Design review of the part built by this model. Coordinates are the model's own, in mm. A direction names the side the tool comes from. Coordinates: 2 decimals unless noted, no trailing zeros. Write each loop counter-clockwise with the first axis right and the second up, starting at its lowest first coordinate (ties: lowest second). Pieces come first, ordered by that corner, then holes.
Q1. Mouldability with a two-part tool opening along Y and no side actions: class faces 1 (the flat face through (-1.6, -9.5, -88.816)), 2 (the flat face through (-1, -15, -104)), 3 (the flat face through (-1, 170, 1)) as pulls with the +Y half, pulls with the -Y half, needs draft (parallel to the pull), parting line crosses it, or undercut.
Q2. For probe 1 along Y at (x, z) = (-41.5, 36); probe 2 along Z at (x, y) = (0, 85.5); probe 3 along Z at (x, y) = (88, -4.5), list the stretches that pass through material, from the lowest coordinate up.
Q3. Take a section at B-B (y = 131). Give the boundary of the cut face in (x, z), and give its area (3 significant figures).
Q4. Take a section at D-D (x = 90.5). Give the boundary of the cut face in (y, z), and give its area (3 significant figures).
Q5. Take a section at C-C (z = 49). Give the boundary of the cut face in (x, y), and give its area (3 significant figures).
Q6. Take a section at A-A (x = 0). Give the boundary of the cut face in (y, z), and give its area (3 significant figures).
Q7. Insertion check: pin 1 (10 mm diameter, centred on x = 46, y = 2.5, fed in from +Z); pin 2 (4 mm diameter, centred on x = -31, y = 138, fed in from -Z); pin 3 (20.5 mm diameter, centred on x = 4.5, z = -101, fed in from -Y). Each pin has a flat end and moves straight along its axis. Give the tip position at first contact, or say it passes through.
Q8. Machinability: for faces 4 (the flat face through (-2, -25, -18)), 5 (the conical face through (40.05, 86.19, 12.61)), 6 (the flat face through (-1, -10, -104)), which of the approach directions +Z, -Z, +X, -X, +Y, -Y give a long, thin tool a straight path to every point of the face, cutting with its end or side? Answer none if there is none.
```python
from build123d import *

# Parameters (mm, degrees)
F0_R     = 45
F1_DEPTH = 170
F1_TAPER = 2
F3_DEPTH = 25
F5_START = -10
F4_R     = 92.5
F5_DEPTH = 5


with BuildPart() as f1:
    # F0 (on Front) → F1 (new body)
    with BuildSketch(Plane.XZ):
        Circle(F0_R)
    extrude(amount=-F1_DEPTH, taper=F1_TAPER)

    # F2 (on face) → F3 (join)
    with BuildSketch(Plane.XZ):
        with BuildLine():
            Line((-114.8654392336, -88.8156135872), (114.8654392336, -88.8156135872))
            ThreePointArc((114.8654392336, -88.8156135872), (0, 89.0399508403), (-114.8654392336, -88.8156135872))
        make_face()
    extrude(amount=F3_DEPTH)

    # F4 (on face) → F5 (join)
    with BuildSketch(Plane.XZ.offset(25).offset(F5_START)):
        with Locations((0, -36.9799211621)):
            Circle(F4_R)
    extrude(amount=-F5_DEPTH)


solid = f1.part
```
Response:
1. face 1: needs draft
1. face 2: pulls with the -Y half
1. face 3: pulls with the +Y half
2. probe 1: y = -25 to 0
2. probe 2: z = -42.01 to 42.01
2. probe 3: z = -88.82 to 53.23
3. outline: circle Ø80.85 at (0, 0)
3. area: 5,130 mm2
4. outline: (-25, -88.82) - (0, -88.82) - (0, 50.72) - (-25, 50.72) - close
4. area: 3,490 mm2
5. outline: (-92.13, -25) - (92.13, -25) - (92.13, 0) - (-92.13, 0) - close
5. area: 4,610 mm2
6. outline: (-25, -88.82) - (-15, -88.82) - (-15, -129.48) - (-10, -129.48) - (-10, -88.82) - (0, -88.82) - (0, -45) - (170, -39.06) - (170, 39.06) - (0, 45) - (0, 89.04) - (-25, 89.04) - close
6. area: 18,900 mm2
7. pin 1: stops at z = 81.95
7. pin 2: stops at z = -27.81
7. pin 3: stops at y = -15
8. face 4: +Z, -Z, +X, -X, -Y
8. face 5: +Y
8. face 6: -Z, +X, -X, +Y
